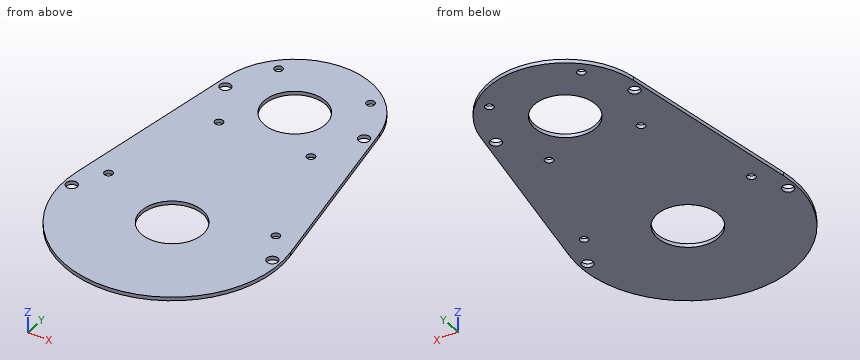
Autodesk Inventor part; units mm, degrees
ref_plane "YZ Plane" through (0, 0, 0) normal (1, 0, 0) x (0, 1, 0)
ref_plane "XZ Plane" through (0, 0, 0) normal (0, 1, 0) x (-1, 0, 0)
ref_plane "XY Plane" through (0, 0, 0) normal (0, 0, 1) x (1, 0, 0)
sketch "Sketch1" plane through (0, 0, 0) normal (0, 0, 1) x (1, 0, 0)
  circle A0 centre (0, 0) radius 52.5 construction
  circle A1 centre (0, 0) radius 25
  circle A2 centre (0, 0) radius 62.5
  line L0 (0, 0) -> (0, 52.5) construction
  line L1 (0, 0) -> (37.1231, 37.1231) construction
  line L2 (0, 0) -> (0, -152.863) construction
  circle A3 centre (0, -152.863) radius 87.5
  line L3 (-86.3219, -138.5528) -> (-61.6585, 10.2216)
  line L4 (86.3219, -138.5528) -> (61.6585, 10.2216)
  circle A4 centre (0, -152.863) radius 25
  circle A5 centre (0, -152.863) radius 81 construction
  circle A6 centre (0, 0) radius 56 construction
  line L5 (0, 0) -> (-56, 0) construction
  line L6 (0, -152.863) -> (-81, -152.863) construction
  dimension "d31" = 162
  dimension "d32" = 112
  dimension "d0" = 105
  dimension "d1" = 50
  dimension "d2" = 125
  dimension "d3" = 45
  dimension "d4" = 152.863
  dimension "d5" = 175
  dimension "d6" = 50
extrude "Extrusion1" add sketch "Sketch1" along normal blind 3
sketch "Sketch2" plane through (0, 0, 0) normal (0, 0, 1) x (1, 0, 0)
  line L0 (0, 0) -> (0, -127.863)
  line L1 (67.5, -127.863) -> (-67.5, -127.863)
  arc A0 (-86.3219, -138.5528) -> (86.3219, -138.5528) centre (0, -152.863) ccw
  dimension "d11" = 127.863
  dimension "d12" = 135
  dimension "d40" = 25
hole "Hole1" at (67.5, -127.863, 0) at (-67.5, -127.863, 0) direction (0, 0, 1) diameter 6.6 end through all
hole "Hole2" at (37.1231, 37.1231, 0) direction (0, 0, 1) diameter 6.6 end through all
pattern_circular "Circular Pattern1" count 4 over 360 about axis through (0, 0, 0) along (0, 0, 1) of "Hole2"
hole "Hole3" at (-56, 0, 0) at (-81, -152.863, 0) direction (0, 0, 1) diameter 9 end through all
mirror "Mirror1" about plane through (0, 0, 0) normal (1, 0, 0) of "Hole3"
properties part number "PWTR-0084" material "Aluminum 6061"
Verification items for the finished model (mm, model axes). Give positions to 0.01 mm unless a question says otherwise; leave off trailing zeros. Order: outer loops, then holes, each group sorted by start corner. A loop starts at its lowest first (then second) coordinate and runs counter-clockwise, first axis right, second up. Notation, with made-up numbers: M -30,46 L 28,46 A12 cw 28,66 Z; hole C -6,-22 d6. An arc over 180 degrees is marked long. Use one line per item in the form item = value. Start each with the question number.
Q1. Section check B-B (y = 0). Enter the section's corners in (x, z), then the cut area to 3 significant figures.
Q2. Section check A-A (x = 0). Enter the section's corners in (y, z), then the cut area to 3 significant figures.
Q3. Section check D-D (z = 1.2). Count the separate pieces of the cut face and the enclosed holes in it, then the cut area to 3 significant figures.
Q4. Section check C-C (x = -81). Enter the section's corners in (y, z), then the cut area to 3 significant figures.
Q5. Scan lines: line 1 along Y through (x, z) = (1, 2.4); line 2 along Y through (x, z) = (0, 1.1); line 3 along X through (y, z) = (2, 2.25). Record each from-to range of solid material in increasing order. Write a range as [from, to].
Q6. Go/stop test with flat-tipped pins: pin 1 Ø1.5 at (y, z) = (5, 1) entering from +X; pin 2 Ø1 at (y, z) = (-155, 1) entering from +X; pin 3 Ø1.5 at (x, z) = (26.5, 1) entering from -Y. Record where each tip stops, or that it passes through.
Evaluation:
q1.outline = M -63.35,0 L -60.5,0 L -60.5,3 L -63.35,3 Z; M -51.5,0 L -25,0 L -25,3 L -51.5,3 Z; M 25,0 L 51.5,0 L 51.5,3 L 25,3 Z; M 60.5,0 L 63.35,0 L 63.35,3 L 60.5,3 Z
q1.area = 176 mm2
q2.outline = M -240.36,0 L -177.86,0 L -177.86,3 L -240.36,3 Z; M -127.86,0 L -25,0 L -25,3 L -127.86,3 Z; M 25,0 L 62.5,0 L 62.5,3 L 25,3 Z
q2.area = 609 mm2
q3.separate_pieces = 1
q3.enclosed_holes = 12
q3.area = 37,000 mm2
q4.outline = M -185.96,0 L -157.36,0 L -157.36,3 L -185.96,3 Z; M -148.36,0 L -106.45,0 L -106.45,3 L -148.36,3 Z
q4.area = 212 mm2
q5.line_1 = [-240.36, -177.84], [-127.88, -24.98], [24.98, 62.49]
q5.line_2 = [-240.36, -177.86], [-127.86, -25], [25, 62.5]
q5.line_3 = [-63.02, -60.03], [-51.97, -24.92], [24.92, 51.97], [60.03, 63.02]
q6.pin_1 = 62.65
q6.pin_2 = 87.48
q6.pin_3 = -236.49
